Input: part model. Units: mm. Frame: model coordinates. Give positions to 0.01 mm unless a question says otherwise; leave off trailing zeros. Loops run counter-clockwise (first coordinate to the right, second up) from the corner with the lowest first, then second, coordinate; pieces in that order, holes last. Notation, with made-up numbers: (71.5, -14.5) - (113.5, -14.5) arc R21 cw to (113.5, 7.5) - close; hole circle Ø9 at (-29, 39.5). An arc over 180 degrees is marked (long way). One line per item, written item: value.
from build123d import *

# Parameters (mm, degrees)
SKETCH1_W            = 120
SKETCH1_H            = 70
BOSS_EXTRUDE1_DEPTH  = 5
BOSS_EXTRUDE4_DEPTH  = 5
BOSS_EXTRUDE5_DEPTH  = 5
BOSS_EXTRUDE7_START  = -70
SKETCH7_R            = 2
BOSS_EXTRUDE7_DEPTH  = 70
SKETCH8_W            = 115.247199032
SKETCH8_H            = 64.754368984
CUT_EXTRUDE1_DEPTH   = 2.5
SKETCH13_W           = 10
SKETCH13_H           = 10
BOSS_EXTRUDE8_DEPTH  = 1
SKETCH14_W           = 10
SKETCH14_H           = 10
BOSS_EXTRUDE9_DEPTH  = 1
SKETCH15_W           = 60
SKETCH15_H           = 10
BOSS_EXTRUDE12_DEPTH = 1
CUT_EXTRUDE2_REACH   = 114.225
CUT_EXTRUDE3_START   = -70
SKETCH17_R           = 1
CUT_EXTRUDE3_DEPTH   = 70
SKETCH18_W           = 60
SKETCH18_H           = 9
BOSS_EXTRUDE15_DEPTH = 1
THICKEN1_START       = 0.540986693
THICKEN1_OUTLINE_W   = 10
THICKEN1_OUTLINE_H   = 8
THICKEN1_DEPTH       = 0.5
THICKEN2_START       = -58.959013307
THICKEN2_OUTLINE_W   = 10
THICKEN2_OUTLINE_H   = 8
THICKEN2_DEPTH       = 0.5
THICKEN3_START       = -58.959013307
THICKEN3_OUTLINE_W   = 10
THICKEN3_OUTLINE_H   = 8
THICKEN3_DEPTH       = 0.5
THICKEN4_START       = 0.540986693
THICKEN4_OUTLINE_W   = 10
THICKEN4_OUTLINE_H   = 8
THICKEN4_DEPTH       = 0.5
SKETCH22_W           = 10
SKETCH22_H           = 1
BOSS_EXTRUDE16_DEPTH = 1
SKETCH23_W           = 10
SKETCH23_H           = 1
BOSS_EXTRUDE17_DEPTH = 1
CUT_EXTRUDE4_DEPTH   = 5
SKETCH28_W           = 10
SKETCH28_H           = 11
BOSS_EXTRUDE18_DEPTH = 8
CUT_EXTRUDE5_START   = -23
SKETCH29_R           = 1
CUT_EXTRUDE5_DEPTH   = 23


# Read off the part's stored shape, not the designer's step: Thicken1, Thicken2, Thicken3, Thicken4
with BuildPart() as part:
    # Sketch1 → Boss-Extrude1 (new body)
    with BuildSketch(Plane(origin=(0, 0, 0), x_dir=(1, 0, 0), z_dir=(0, 1, 0))):
        Rectangle(SKETCH1_W, SKETCH1_H)
    extrude(amount=BOSS_EXTRUDE1_DEPTH)

    # Sketch2 → Boss-Extrude4 (add)
    with BuildSketch(Plane(origin=(0, 0, -35), x_dir=(-1, 0, 0), z_dir=(0, 0, -1))):
        Polygon((74.508152461, 38.345236523), (58.959013307, 5), (60, 5), (60, -0.000631219), (61.04069235, -0.000631219), (78.133383609, 36.654763477), align=None)
    extrude(amount=-BOSS_EXTRUDE4_DEPTH)

    # Sketch6 → Boss-Extrude5 (add)
    with BuildSketch(Plane.XY.offset(35)):
        Polygon((-61.04069235, -0.000631219), (-60, 0), (-60, 5), (-58.959013307, 5), (-74.508152461, 38.345236523), (-78.133383609, 36.654763477), align=None)
    extrude(amount=-BOSS_EXTRUDE5_DEPTH)

    # Sketch7 → Boss-Extrude7 (add)
    with BuildSketch(Plane(origin=(0, 0, -35), x_dir=(-1, 0, 0), z_dir=(0, 0, -1)).offset(BOSS_EXTRUDE7_START)):
        with Locations(Location((76.320768035, 37.5, 0), (0, 0, 335))):
            Circle(SKETCH7_R)
    extrude(amount=BOSS_EXTRUDE7_DEPTH)

    # Sketch8 → Cut-Extrude1 (cut)
    with BuildSketch(Plane(origin=(0, 5, 0), x_dir=(1, 0, 0), z_dir=(0, 1, 0))):
        Rectangle(SKETCH8_W, SKETCH8_H)
    extrude(amount=-CUT_EXTRUDE1_DEPTH, mode=Mode.SUBTRACT)

    # Sketch13 → Boss-Extrude8 (add)
    with BuildSketch(Plane(origin=(0, 0, -35), x_dir=(-1, 0, 0), z_dir=(0, 0, -1))):
        with Locations((-55, -5)):
            Rectangle(SKETCH13_W, SKETCH13_H)
    extrude(amount=-BOSS_EXTRUDE8_DEPTH)

    # Sketch14 → Boss-Extrude9 (add)
    with BuildSketch(Plane.XY.offset(35)):
        with Locations((55, -5)):
            Rectangle(SKETCH14_W, SKETCH14_H)
    extrude(amount=-BOSS_EXTRUDE9_DEPTH)

    # Sketch15 → Boss-Extrude12 (add)
    with BuildSketch(Plane(origin=(0, 0, -35), x_dir=(-1, 0, 0), z_dir=(0, 0, -1))):
        with Locations((28.959013307, -5)):
            Rectangle(SKETCH15_W, SKETCH15_H)
    boss_extrude12 = extrude(amount=-BOSS_EXTRUDE12_DEPTH)

    # Mirror1: Boss-Extrude12 across plane
    add(boss_extrude12.mirror(Plane.XY))

    # Cut-Extrude2: up to this face of the body (flat: up to its plane)
    cut_extrude2_end = Plane(part.part.faces().sort_by_distance((-15.670325555, 0.904669602, 35))[0])
    # Sketch16 → Cut-Extrude2 (cut, up to the picked face)
    with BuildSketch(Plane(origin=(0, 0, -35), x_dir=(-1, 0, 0), z_dir=(0, 0, -1)), mode=Mode.PRIVATE) as cut_extrude2_sk1:
        with BuildLine():
            Line((3.959013307, -4), (53.959013307, -4))
            ThreePointArc((53.959013307, -4), (54.959013307, -5), (53.959013307, -6))
            Line((53.959013307, -6), (3.959013307, -6))
            ThreePointArc((3.959013307, -6), (2.959013307, -5), (3.959013307, -4))
        make_face()
    cut_extrude2_tool1 = split(extrude(cut_extrude2_sk1.sketch, amount=-CUT_EXTRUDE2_REACH, mode=Mode.PRIVATE), bisect_by=cut_extrude2_end, keep=Keep.BOTH, mode=Mode.PRIVATE)
    add(cut_extrude2_tool1.solids().sort_by(Axis((-28.959013, -5, -35), (0, 0, 1)))[0], mode=Mode.SUBTRACT)

    # Sketch17 → Cut-Extrude3 (cut)
    with BuildSketch(Plane(origin=(0, 0, -35), x_dir=(-1, 0, 0), z_dir=(0, 0, -1)).offset(CUT_EXTRUDE3_START)):
        with Locations((-55, -5)):
            Circle(SKETCH17_R)
    extrude(amount=CUT_EXTRUDE3_DEPTH, mode=Mode.SUBTRACT)

    # Sketch18 → Boss-Extrude15 (add)
    with BuildSketch(Plane.XZ.offset(10)):
        with Locations((-28.959013307, 30.5)):
            Rectangle(SKETCH18_W, SKETCH18_H)
        with Locations((-28.959013307, -30.5)):
            Rectangle(SKETCH18_W, SKETCH18_H)
    extrude(amount=BOSS_EXTRUDE15_DEPTH)

    # Thicken1 outline → Thicken1 (add)
    with BuildSketch(Plane.YZ.offset(THICKEN1_START)):
        with Locations((-5, 30)):
            Rectangle(THICKEN1_OUTLINE_W, THICKEN1_OUTLINE_H)
    extrude(amount=THICKEN1_DEPTH)

    # Thicken2 outline → Thicken2 (add)
    with BuildSketch(Plane.YZ.offset(THICKEN2_START)):
        with Locations((-5, -30)):
            Rectangle(THICKEN2_OUTLINE_W, THICKEN2_OUTLINE_H)
    extrude(amount=THICKEN2_DEPTH)

    # Thicken3 outline → Thicken3 (add)
    with BuildSketch(Plane.YZ.offset(THICKEN3_START)):
        with Locations((-5, 30)):
            Rectangle(THICKEN3_OUTLINE_W, THICKEN3_OUTLINE_H)
    extrude(amount=THICKEN3_DEPTH)

    # Thicken4 outline → Thicken4 (add)
    with BuildSketch(Plane.YZ.offset(THICKEN4_START)):
        with Locations((-5, -30)):
            Rectangle(THICKEN4_OUTLINE_W, THICKEN4_OUTLINE_H)
    extrude(amount=THICKEN4_DEPTH)

    # Sketch22 → Boss-Extrude16 (add)
    with BuildSketch(Plane.XY.offset(35)):
        with Locations((55, -10.5)):
            Rectangle(SKETCH22_W, SKETCH22_H)
    extrude(amount=-BOSS_EXTRUDE16_DEPTH)

    # Sketch23 → Boss-Extrude17 (add)
    with BuildSketch(Plane(origin=(0, 0, -35), x_dir=(-1, 0, 0), z_dir=(0, 0, -1))):
        with Locations((-55, -10.5)):
            Rectangle(SKETCH23_W, SKETCH23_H)
    extrude(amount=-BOSS_EXTRUDE17_DEPTH)

    # Sketch25 → Cut-Extrude4 (cut)
    with BuildSketch(Plane.XZ.offset(11)):
        with BuildLine():
            Line((-2.866454916, 32.5), (-54.996437016, 32.5))
            ThreePointArc((-54.996437016, 32.5), (-56.996437016, 30.5), (-54.996437016, 28.5))
            Line((-54.996437016, 28.5), (-2.866454916, 28.5))
            ThreePointArc((-2.866454916, 28.5), (-0.866454916, 30.5), (-2.866454916, 32.5))
        make_face()
        with BuildLine():
            Line((-2.866454916, -28.5), (-54.996437016, -28.5))
            ThreePointArc((-54.996437016, -28.5), (-56.996437016, -30.5), (-54.996437016, -32.5))
            Line((-54.996437016, -32.5), (-2.866454916, -32.5))
            ThreePointArc((-2.866454916, -32.5), (-0.866454916, -30.5), (-2.866454916, -28.5))
        make_face()
    extrude(amount=-CUT_EXTRUDE4_DEPTH, mode=Mode.SUBTRACT)

    # Sketch28 → Boss-Extrude18 (add)
    with BuildSketch(Plane(origin=(0, 0, -35), x_dir=(-1, 0, 0), z_dir=(0, 0, -1))):
        with Locations((-55, -5.5)):
            Rectangle(SKETCH28_W, SKETCH28_H)
    extrude(amount=-BOSS_EXTRUDE18_DEPTH)

    # Sketch29 → Cut-Extrude5 (cut)
    with BuildSketch(Plane(origin=(0, 0, -35), x_dir=(-1, 0, 0), z_dir=(0, 0, -1)).offset(CUT_EXTRUDE5_START)):
        with Locations((-55, -5)):
            Circle(SKETCH29_R)
    extrude(amount=CUT_EXTRUDE5_DEPTH, mode=Mode.SUBTRACT)


solid = part.part
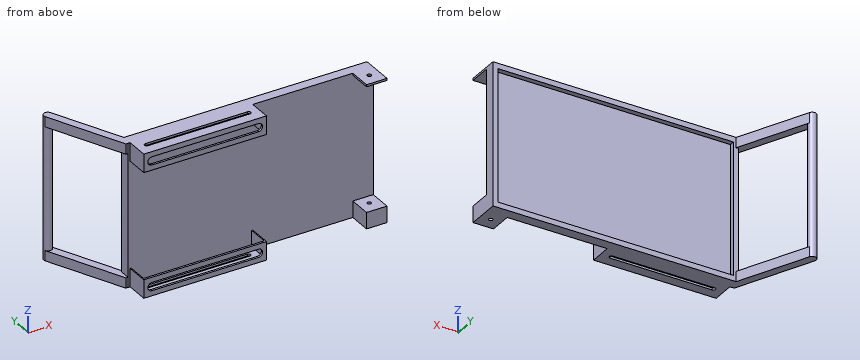
Item 1: Section C-C, the plane y = 28. Output: boundary loops of the cut face in (x, z), and give its area (3 significant figures).
Verdict:
outline: (-74.1, -35) - (-69.68, -35) - (-69.68, -30) - (-74.1, -30) - close; (-74.1, 30) - (-69.68, 30) - (-69.68, 35) - (-74.1, 35) - close
area: 44.1 mm^2
Item 2: Section A-A, the plane z = -12.5. Output: boundary loops of the cut face in (x, y).
Verdict:
outline: circle Ø4 at (-76.32, 37.5); (-60, 0) - (60, 0) - (60, 5) - (57.62, 5) - (57.62, 2.5) - (-57.62, 2.5) - (-57.62, 5) - (-60, 5) - close
Item 3: Section B-B, the plane x = 46. Output: boundary loops of the cut face in (y, z), and give its area (3 significant figures).
Verdict:
outline: (0, -35) - (5, -35) - (5, -32.38) - (2.5, -32.38) - (2.5, 32.38) - (5, 32.38) - (5, 35) - (0, 35) - close
area: 188 mm^2
Item 4: Material intervals for L1, parallel to X at y = -5, z = 34.75; L2, parallel to X at y = -5, z = -29; L3, parallel to Y at x = 55, z = 34.7, sorted ascending.
Verdict:
L1: x = -58.96 to -54.96, -2.96 to 1.04, 50 to 54, 56 to 60
L2: x = -58.96 to -58.46, 0.54 to 1.04, 50 to 54, 56 to 60
L3: y = -11 to -6, -4 to 5
Item 5: Pin query (flat end, axial travel): P1, Ø10, axis at x = -50, z = 25.5, coming from the +Y side; P2, Ø1.1, axis at y = -4, z = 34.5, coming from the -X side; P3, Ø1.8, axis at x = 55, y = -5, coming from the -Z side; P4, Ø7, axis at y = -3, z = -32, coming from the -X side. Return the tip coordinate at first contact, or that it passes through.
Verdict:
P1: stops at y = 2.5
P2: stops at x = -58.96
P3: passes through
P4: stops at x = -61.27
